Build history of the part. All positions in model axes, mm. Face numbers are marked on the shaded views. A direction names the side the tool comes from. Round coordinates to 2 decimals unless told otherwise and drop trailing zeros. Loops run counter-clockwise (first coordinate to the right, second up) from the corner with the lowest first, then second, coordinate; pieces in that order, holes last. Notation, with made-up numbers: (55, 12.25) - (63, 12.25) arc R29 ccw to (63, 44.25) - close; hole circle Ø9 at (46, -26.5). An arc over 180 degrees is marked (long way). Answer as CSV lines item,"result". Start each with the question number.
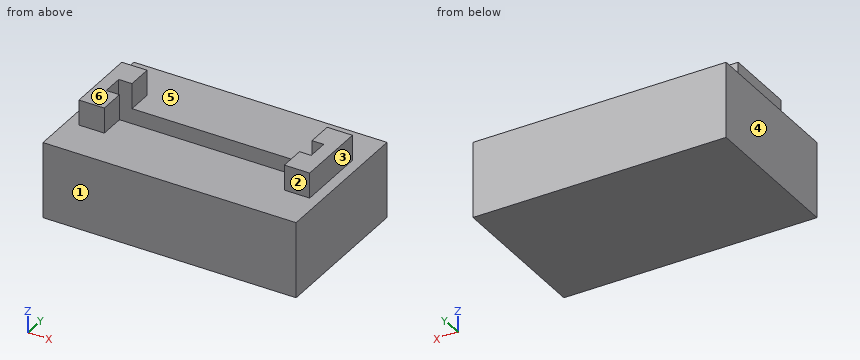
```python
from build123d import *

# Parameters (mm, degrees)
F1_DEPTH = 5
F0_W     = 50
F0_H     = 30
F2_DEPTH = 15
F3_DEPTH = 20


with BuildPart() as f1:
    # F0 (on Top) → F1 (new body)
    with BuildSketch(Plane.XY):
        Polygon((17.932241, -2.0625), (20.25, -2.0625), (20.25, 2.0625), (17.932241, 2.0625), (-17.639818, 2.0625), (-20.25, 2.0625), (-20.25, -2.0625), (-17.639818, -2.0625), align=None)
    extrude(amount=F1_DEPTH)

    # F0 (on Top) → F2 (join)
    with BuildSketch(Plane.XY):
        Rectangle(F0_W, F0_H)
        Polygon((17.932241, -7.0625), (17.932241, -2.0625), (-17.639818, -2.0625), (-17.639818, -7.0625), (-22.639818, -7.0625), (-22.639818, 7.0625), (-17.639818, 7.0625), (-17.639818, 2.0625), (17.932241, 2.0625), (17.932241, 7.0625), (22.932241, 7.0625), (22.932241, -7.0625), align=None, mode=Mode.SUBTRACT)
    extrude(amount=F2_DEPTH)

    # F0 (on Top) → F3 (join)
    with BuildSketch(Plane.XY):
        Polygon((-17.639818, -7.0625), (-17.639818, -2.0625), (-20.25, -2.0625), (-20.25, 2.0625), (-17.639818, 2.0625), (-17.639818, 7.0625), (-22.639818, 7.0625), (-22.639818, -7.0625), align=None)
        Polygon((20.25, 2.0625), (20.25, -2.0625), (17.932241, -2.0625), (17.932241, -7.0625), (22.932241, -7.0625), (22.932241, 7.0625), (17.932241, 7.0625), (17.932241, 2.0625), align=None)
    extrude(amount=F3_DEPTH)


solid = f1.part
```
Q1. Pin check, flat tips, straight feed: pin 1 Ø1.5 at (y, z) = (3, 16.5) entering from +X; pin 2 Ø2.5 at (x, z) = (-19, 16.5) entering from -Y; pin 3 Ø2.5 at (x, z) = (-19.5, 18) entering from +Y. Stop position of each tip, or through.
Q2. Band-saw the part on C-C, the plane y = 3.75. List the corners of the cut face in (x, z), then the cut area to 3 significant figures.
Q3. Tool access for the marked faces 1 and 2: list every direction of +Z, -Z, +X, -X, +Y, -Y with a clear straight run to the whole face (end or side of a thin tool).
Q4. Band-saw the part on D-D, the plane x = -11.5. List the corners of the cut face in (y, z).
Q5. Wall check: probe 1 along Y at (x, z) = (-4, 8); probe 2 along X at (y, z) = (-3, 18.75); probe 3 along Z at (x, y) = (-17, -8.5). Give the ranges that are in metal, low to high. Write a range as [from, to].
Q6. Band-saw the part on A-A, the plane z = 19. List the corners of the cut face in (x, y), then the cut area to 3 significant figures.
Q7. Band-saw the part on B-B, the plane z = 14.5. List the corners of the cut face in (x, y), then the cut area to 3 significant figures.
Q8. Two-plate mould, pull along X, no slides. Class the marked faces 3, 4, 5 and 6: released by +X, released by -X, zero draft, split by the parting line, or undercut.
Reported:
1,pin 1,"stops at x = 22.93"
1,pin 2,"stops at y = -7.06"
1,pin 3,"stops at y = 7.06"
2,outline,"(-25, 0) - (25, 0) - (25, 15) - (22.93, 15) - (22.93, 20) - (17.93, 20) - (17.93, 15) - (-17.64, 15) - (-17.64, 20) - (-22.64, 20) - (-22.64, 15) - (-25, 15) - close"
2,area,"800 mm2"
3,face 1,"+Z, -Z, +X, -X, -Y"
3,face 2,"+Z, +X, -X, -Y"
4,outline,"(-15, 0) - (15, 0) - (15, 15) - (2.06, 15) - (2.06, 5) - (-2.06, 5) - (-2.06, 15) - (-15, 15) - close"
5,probe 1,"y = [-15, -2.06], [2.06, 15]"
5,probe 2,"x = [-22.64, -17.64], [17.93, 22.93]"
5,probe 3,"z = [0, 15]"
6,outline,"(-22.64, -7.06) - (-17.64, -7.06) - (-17.64, -2.06) - (-20.25, -2.06) - (-20.25, 2.06) - (-17.64, 2.06) - (-17.64, 7.06) - (-22.64, 7.06) - close; (17.93, -7.06) - (22.93, -7.06) - (22.93, 7.06) - (17.93, 7.06) - (17.93, 2.06) - (20.25, 2.06) - (20.25, -2.06) - (17.93, -2.06) - close"
6,area,"121 mm2"
7,outline,"(-25, -15) - (25, -15) - (25, 15) - (-25, 15) - close; hole (-20.25, -2.06) - (20.25, -2.06) - (20.25, 2.06) - (-20.25, 2.06) - close"
7,area,"1,330 mm2"
8,face 3,"released by +X"
8,face 4,"released by -X"
8,face 5,"undercut"
8,face 6,"zero draft"
